Work out the finished part from the listing and answer in its coordinate system (mm). Face numbers are marked on the shaded views. A direction names the side the tool comes from. Give positions to 0.01 mm unless a question says otherwise; leave off trailing zeros. Order: outer loops, then holes, each group sorted by start corner. A loop starts at its lowest first (then second) coordinate and runs counter-clockwise, first axis right, second up. Notation, with made-up numbers: (20, 71) - (77, 71) arc R30 cw to (77, 97) - close; hole circle Ø4 at (66, 4.25). An arc over 180 degrees is marked (long way). Return JSON: item names as keys, results as strings. Group by question number.
from build123d import *

# Parameters (mm, degrees)
F0_W     = 52.5068640709
F0_H     = 35.3771150112
F1_DEPTH = 330
F2_DEPTH = 600
F3_DEPTH = 600
F4_T     = -18


with BuildPart() as f1:
    # F0 (on Front) → F1 (new body)
    with BuildSketch(Plane.XZ):
        with Locations((-26.2534320354, 17.6885575056)):
            Rectangle(F0_W, F0_H)
    extrude(amount=-F1_DEPTH)

    # F2 (add): a face of the model
    f2_faces = [f1.faces().sort_by_distance(p)[0] for p in [
        (-26.2534320354, 165, 0),
    ]]
    extrude(f2_faces, amount=-F2_DEPTH)

    # F3 (add): a face of the model
    f3_faces = [f1.faces().sort_by_distance(p)[0] for p in [
        (0, 165, 300),
    ]]
    extrude(f3_faces, amount=-F3_DEPTH)

    # F4
    f4_openings = [f1.faces().sort_by_distance(p)[0] for p in [
        (-300, 330, 300),
    ]]
    offset(amount=F4_T, openings=f4_openings)


solid = f1.part
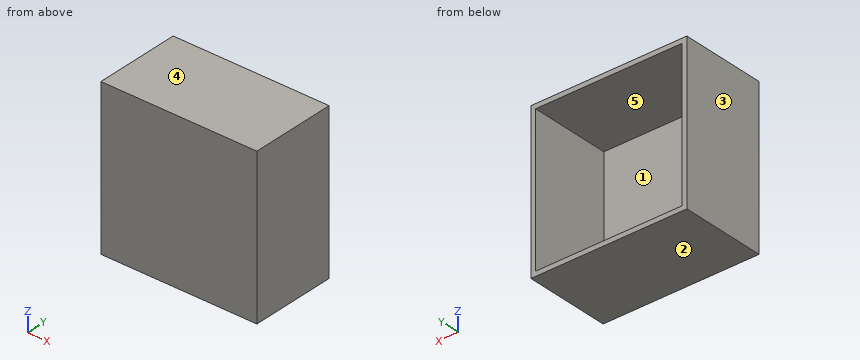
1. Each of these flat-tipped pins is pushed along its axis until it touches: pin 1 (12 mm diameter, centred on x = -200, y = 169, fed in from -Z); pin 2 (2 mm diameter, centred on x = -477, z = 283.5, fed in from +Y). Where does it stop, or does it pass through?
2. The part is cut by section A-A (y = 141.5). Give the vertices of the cut face in (x, z), and give its area (3 significant figures).
3. The part is cut by section C-C (x = -76.5). Give the vertices of the cut face in (y, z).
4. The part is cut by section B-B (z = 360.5). Give the vertices of the cut face in (x, y), and give its area (3 significant figures).
5. Determine the mould class of the marked faces 1, 2 and 3 for opening direction Z: released by +Z, released by -Z, zero draft, split by the parting line, or undercut.
6. Consider probe 1 along Z at (x, y) = (-411, 27); probe 2 along X at (y, z) = (252.5, 485); probe 3 along Y at (x, z) = (-438, 211.5). Determine where each line is inside the solid, lowest interval first. Write a range as from..to.
7. A tool of negligible diameter and unlimited length cuts with its end or side. For the marked faces 4 and 5, from which of +Z, -Z, +X, -X, +Y, -Y can it reach the whole face along a straight path? Write none if from no direction.
Answers:
{
 "1": {"pin 1": "stops at z = 0", "pin 2": "stops at y = 18"},
 "2": {"outline": "(-600, 0) - (0, 0) - (0, 600) - (-600, 600) - close; hole (-582, 18) - (-18, 18) - (-18, 582) - (-582, 582) - close", "area": "41,900 mm^2"},
 "3": {"outline": "(0, 0) - (330, 0) - (330, 18) - (18, 18) - (18, 582) - (330, 582) - (330, 600) - (0, 600) - close"},
 "4": {"outline": "(-600, 0) - (0, 0) - (0, 330) - (-18, 330) - (-18, 18) - (-582, 18) - (-582, 330) - (-600, 330) - close", "area": "22,000 mm^2"},
 "5": {"face 1": "undercut", "face 2": "released by -Z", "face 3": "zero draft"},
 "6": {"probe 1": "z = 0..18, 582..600", "probe 2": "x = -600..-582, -18..0", "probe 3": "y = 0..18"},
 "7": {"face 4": "+Z, +X, -X, +Y, -Y", "face 5": "+Y"}
}
